Autodesk Inventor part; units mm, degrees
ref_plane "YZ Plane" through (0, 0, 0) normal (1, 0, 0) x (0, 1, 0)
ref_plane "XZ Plane" through (0, 0, 0) normal (0, 1, 0) x (-1, 0, 0)
ref_plane "XY Plane" through (0, 0, 0) normal (0, 0, 1) x (1, 0, 0)
sketch "Sketch1" plane through (0, 0, 0) normal (0, 0, 1) x (1, 0, 0)
  line L0 (-8, 32) -> (8, 32)
  line L1 (8, 32) -> (8, -32)
  line L2 (8, -32) -> (-8, -32)
  line L3 (-8, -32) -> (-8, 32)
  point P0 (0, 0)
  dimension "d0" = 16
  dimension "d1" = 64
  dimension "d2" = 8
  dimension "d3" = 32
extrude "Extrusion1" add sketch "Sketch1" along normal blind 3.2
shell "Shell1" thickness 1.5 removed faces 1 at (-2.6667, 10.6667, 0)
sketch "Sketch2" plane through (0, 0, 3.2) normal (0, 0, 1) x (1, 0, 0)
  circle A0 centre (4, -28) radius 2.5
  line L0 (8, 32) -> (8, -32)
  line L1 (8, -32) -> (-8, -32)
  dimension "d7" = 5
  dimension "d10" = 4
  dimension "d11" = 4
extrude "Extrusion2" add sketch "Sketch2" along normal blind 1.6
sketch "Sketch3" plane through (6.5, -30.5, 1.7) normal (0, 0, -1) x (-1, 0, 0)
  circle A0 centre (2.5, 2.5) radius 2.5
  circle A1 centre (2.5, 2.5) radius 1.2
  point P0 (6.5, 30.5)
  dimension "d18" = 2.4
extrude "Extrusion3" cut sketch "Sketch3" against normal blind 1.6 contours A1
pattern_linear "Rectangular Pattern1" count 8 spacing 8 along (0, 1, 0) count 2 spacing 8 along (-1, 0, 0) of "Extrusion2", "Extrusion3"
sketch "Sketch4" plane through (6.5, -30.5, 1.7) normal (0, 0, -1) x (-1, 0, 0)
  circle A0 centre (2.5, 10.5) radius 1.2
  circle A1 centre (2.5, 2.5) radius 1.2
  line L0 (0, 61) -> (0, 0)
  line L1 (0, 0) -> (13, 0)
  circle A2 centre (6.5, 6.5) radius 3.15
  circle A3 centre (6.5, 6.5) radius 2.5
  point P0 (6.5, 30.5)
  dimension "d21" = 6.5
  dimension "d22" = 6.5
  dimension "d23" = 10.5
  dimension "d24" = 2.5
  dimension "d25" = 5
  dimension "d26" = 6.3
extrude "Extrusion4" add sketch "Sketch4" along normal up to surface (1.7 mm away) contours A2
pattern_linear "Rectangular Pattern2" count 7 spacing 8 along (0, 1, 0) of "Extrusion4"
equation "\"d0\" = 0.8 * WIDTH"
equation "\"d1\" = 0.8 * LENGTH"
equation "\"d4\" = HEIGHT"
equation "\"d21\" = 0.5 * d23 + 0.5 * d24"
equation "\"d22\" = d21"
equation "\"WIDTH\" = 2"
equation "\"HEIGHT\" = 3.2"
properties part number "3034" material "Steel"
Geometry: final body of the model. Coordinates: model frame, mm. A direction names the side the tool comes from. Round coordinates to 2 decimals unless told otherwise and drop trailing zeros. Write each loop counter-clockwise with the first axis right and the second up, starting at its lowest first coordinate (ties: lowest second). Pieces come first, ordered by that corner, then holes. Notation, with made-up numbers: (35.25, 12) -> (69.25, 12) arc R22 ccw to (69.25, 42) -> close; hole circle Ø2 at (64, 74.25). An arc over 180 degrees is marked (long way). Return JSON: item names as keys, results as strings.
Q1. Section A-A on y = 12. Return the cut outline in (x, z).
From the geometry:
{"outline": "(-8, 0) -> (-6.5, 0) -> (-6.5, 1.7) -> (-5.2, 1.7) -> (-5.2, 3.3) -> (-2.8, 3.3) -> (-2.8, 1.7) -> (2.8, 1.7) -> (2.8, 3.3) -> (5.2, 3.3) -> (5.2, 1.7) -> (6.5, 1.7) -> (6.5, 0) -> (8, 0) -> (8, 3.2) -> (6.5, 3.2) -> (6.5, 4.8) -> (1.5, 4.8) -> (1.5, 3.2) -> (-1.5, 3.2) -> (-1.5, 4.8) -> (-6.5, 4.8) -> (-6.5, 3.2) -> (-8, 3.2) -> close"}
Q2. First-contact query: pin 1 Ø1 at (y, z) = (-6, 4) entering from -X; pin 2 Ø1.4 at (x, y) = (-4, 4) entering from -Z; pin 3 Ø3 at (x, y) = (4, -28) entering from -Z. Flat tips, straight axial feed; report the tip coordinate or a pass-through.
From the geometry:
{"pin 1": "x = -6", "pin 2": "z = 3.3", "pin 3": "z = 1.7"}
Q3. Set-up query: faces 3 (the cylindrical face through (6.385, 3.249, 3.989)), 4 (the flat face through (4, 0, 1.7)), 5 (the flat face through (-7, 7, 0)). Return all of +Z, -Z, +X, -X, +Y, -Y with unobstructed straight access to the full face (end or side cutting, diameter ignored); none if empty.
From the geometry:
{"face 3": "+Z", "face 4": "-Z", "face 5": "-Z, +X, -X, +Y, -Y"}
Q4. Ray query, line 1 (Y direction, x = 3.5, z = 1.5); line 2 (Z direction, x = 3.25, y = -28); line 3 (Z direction, x = -1.75, y = -6). Return the intervals inside material, ascending.
From the geometry:
{"line 1": "-32 to -30.5, 30.5 to 32", "line 2": "3.3 to 4.8", "line 3": "0 to 3.2"}
Q5. Mould query, pull axis Y, two halves, no side actions, for faces 1 (the cylindrical face through (0.41, 4.877, 0.862)), 2 (the flat face through (4, 4, 4.8)). Classes: +Y half, -Y half, draft (parallel to the pull), parting line (faces both ways), or undercut.
From the geometry:
{"face 1": "undercut", "face 2": "draft"}
Q6. Section B-B on y = -8. Return the cut outline in (x, z).
From the geometry:
{"outline": "(-8, 0) -> (-6.5, 0) -> (-6.5, 1.7) -> (-3.15, 1.7) -> (-3.15, 0) -> (-2.5, 0) -> (-2.5, 1.7) -> (2.5, 1.7) -> (2.5, 0) -> (3.15, 0) -> (3.15, 1.7) -> (6.5, 1.7) -> (6.5, 0) -> (8, 0) -> (8, 3.2) -> (-8, 3.2) -> close"}
